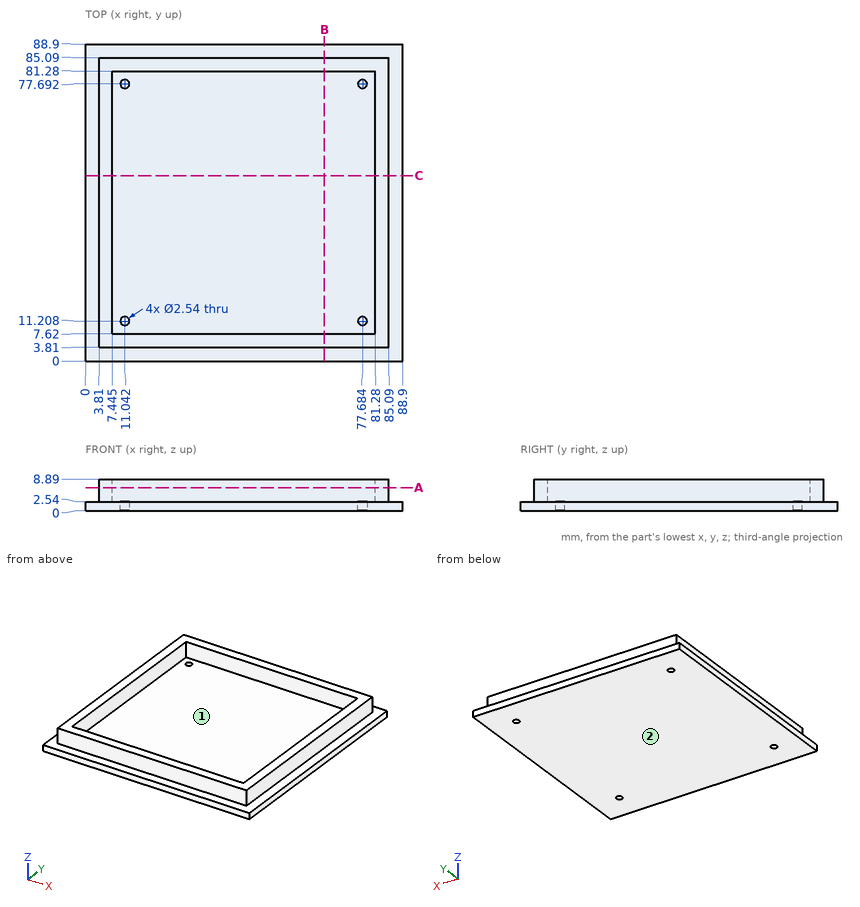
The figure shows three views and two pictorial views of one solid part (mm, origin at its lowest corner). Answer the questions. Round coordinates to 2 decimals unless told otherwise and drop trailing zeros. Loops run counter-clockwise (first coordinate to the right, second up) from the corner with the lowest first, then second, coordinate; pieces in that order, holes last. Notation, with made-up numbers: M -20.75,17 L 31.25,17 A26 cw 31.25,47 Z; hole C 89,1.25 d5. An arc over 180 degrees is marked long. Use CSV: the item, a comma, the result in double quotes.
Q1. Section C-C, the plane y = 52 is taken. Determine the outline of the cut face in (x, z) (1 decimal).
Determined:
outline,"M 0,0 L 88.9,0 L 88.9,2.5 L 85.1,2.5 L 85.1,8.9 L 81.3,8.9 L 81.3,2.5 L 7.4,2.5 L 7.4,8.9 L 3.8,8.9 L 3.8,2.5 L 0,2.5 Z"
Q2. Section B-B, the plane x = 67 is taken. Determine the outline of the cut face in (y, z).
Determined:
outline,"M 0,0 L 88.9,0 L 88.9,2.54 L 85.09,2.54 L 85.09,8.89 L 81.28,8.89 L 81.28,2.54 L 7.62,2.54 L 7.62,8.89 L 3.81,8.89 L 3.81,2.54 L 0,2.54 Z"
Q3. Each of these flat-tipped pins is pushed along its axis until it touches: pin 1 (1.9 mm diameter, centred on x = 51, z = 4.5, fed in from -Y); pin 2 (1.9 mm diameter, centred on x = 55.5, z = 5.5, fed in from +Y); pin 3 (5 mm diameter, centred on x = 18, y = 64, fed in from +Z). Where does it stop, or does it pass through?
Determined:
pin 1,"y = 3.81"
pin 2,"y = 85.09"
pin 3,"z = 2.54"
Q4. The mould has two halves that part along X. Classify the marked faces 1 and 2: pulls with the +X half, pulls with the -X half, needs draft (parallel to the pull), parting line crosses it, or undercut.
Determined:
face 1,"undercut"
face 2,"needs draft"
Q5. Consider L1, parallel to Y at x = 21, z = 7.75; L2, parallel to X at y = 59, z = 3.5 (1 decimal); L3, parallel to Z at x = 58, y = 61. Determine where each line is inside the solid, lowest interval first.
Determined:
L1,"3.81 to 7.62, 81.28 to 85.09"
L2,"3.8 to 7.4, 81.3 to 85.1"
L3,"0 to 2.54"
Q6. Section A-A, the plane z = 6.5 is taken. Determine the outline of the cut face in (x, y) (1 decimal), then the cut area to 3 significant figures.
Determined:
outline,"M 3.8,3.8 L 85.1,3.8 L 85.1,85.1 L 3.8,85.1 Z; hole M 7.4,7.6 L 81.3,7.6 L 81.3,81.3 L 7.4,81.3 Z"
area,"1,170 mm2"
